from build123d import *

# Parameters (mm, degrees)
F1_DEPTH = 762
F2_R     = 5
F3_DEPTH = 25
F4_R     = 5
F5_DEPTH = 25
F6_R     = 5
F7_DEPTH = 25
F8_R     = 5
F9_DEPTH = 25


with BuildPart() as f1:
    # F0 (on Front) → F1 (new body)
    with BuildSketch(Plane.XZ):
        with BuildLine():
            Line((20.354675, 24.193632), (-17.745325, 24.193632))
            ThreePointArc((-17.745325, 24.193632), (-22.235453, 22.33376), (-24.095325, 17.843632))
            Line((-24.095325, 17.843632), (-24.095325, -20.256368))
            ThreePointArc((-24.095325, -20.256368), (-22.235453, -24.746497), (-17.745325, -26.606368))
            Line((-17.745325, -26.606368), (20.354675, -26.606368))
            ThreePointArc((20.354675, -26.606368), (24.844803, -24.746497), (26.704675, -20.256368))
            Line((26.704675, -20.256368), (26.704675, 17.843632))
            ThreePointArc((26.704675, 17.843632), (24.844803, 22.33376), (20.354675, 24.193632))
        make_face()
        with BuildLine():
            ThreePointArc((-17.745325, 11.493632), (-15.885453, 15.98376), (-11.395325, 17.843632))
            Line((-11.395325, 17.843632), (14.004675, 17.843632))
            ThreePointArc((14.004675, 17.843632), (18.494803, 15.98376), (20.354675, 11.493632))
            Line((20.354675, 11.493632), (20.354675, -13.906368))
            ThreePointArc((20.354675, -13.906368), (18.494803, -18.396497), (14.004675, -20.256368))
            Line((14.004675, -20.256368), (-11.395325, -20.256368))
            ThreePointArc((-11.395325, -20.256368), (-15.885453, -18.396497), (-17.745325, -13.906368))
            Line((-17.745325, -13.906368), (-17.745325, 11.493632))
        make_face(mode=Mode.SUBTRACT)
    extrude(amount=F1_DEPTH)

    # F2 (on face) → F3 (cut)
    with BuildSketch(Plane.YZ.offset(26.704675)):
        with Locations((-15, 9.193632)):
            Circle(F2_R)
        with Locations((-15, -11.606368)):
            Circle(F2_R)
        with Locations((-61.2, 9.193632)):
            Circle(F2_R)
        with Locations((-61.2, -11.606368)):
            Circle(F2_R)
    extrude(amount=-F3_DEPTH, mode=Mode.SUBTRACT)

    # F4 (on face) → F5 (cut)
    with BuildSketch(Plane(origin=(0, 0, -26.606368), x_dir=(1, 0, 0), z_dir=(0, 0, -1))):
        with Locations((11.704675, 15)):
            Circle(F4_R)
        with Locations((-9.095325, 15)):
            Circle(F4_R)
        with Locations((11.704675, 61.2)):
            Circle(F4_R)
        with Locations((-9.095325, 61.2)):
            Circle(F4_R)
    extrude(amount=-F5_DEPTH, mode=Mode.SUBTRACT)

    # F6 (on face) → F7 (cut)
    with BuildSketch(Plane(origin=(0, 0, -26.606368), x_dir=(1, 0, 0), z_dir=(0, 0, -1))):
        with Locations((1.304675, 738.9)):
            Circle(F6_R)
        with Locations((1.304675, 708.9)):
            Circle(F6_R)
    extrude(amount=-F7_DEPTH, mode=Mode.SUBTRACT)

    # F8 (on face) → F9 (cut)
    with BuildSketch(Plane.YZ.offset(26.704675)):
        with Locations((-738.9, -1.206368)):
            Circle(F8_R)
        with Locations((-708.9, -1.206368)):
            Circle(F8_R)
    extrude(amount=-F9_DEPTH, mode=Mode.SUBTRACT)


solid = f1.part
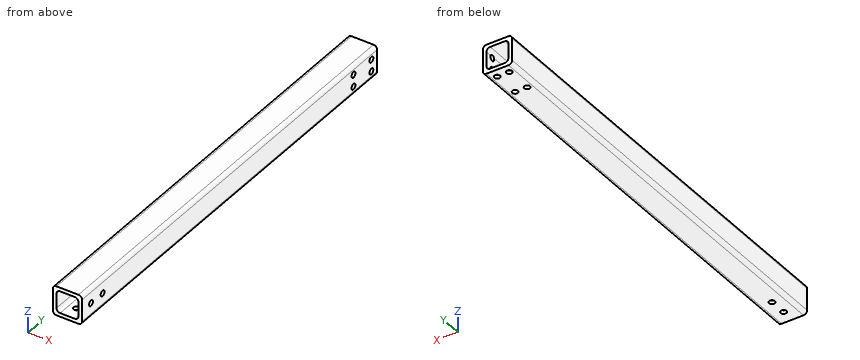
Check sheet for the modelled part. Datum: model origin and axes. Units: mm. Give positions to 0.01 mm unless a question says otherwise; leave off trailing zeros. Write each loop counter-clockwise with the first axis right and the second up, starting at its lowest first coordinate (ties: lowest second). Pieces come first, ordered by that corner, then holes. Notation, with made-up numbers: (36, 47.5) -> (83, 47.5) arc R20 cw to (83, 56.5) -> close; hole circle Ø10 at (0.5, -14.5). An arc over 180 degrees is marked (long way). One line per item, written item: value. Start each with the question number.
Item 1: Gauge pin test, flat end, axial feed: pin 1 (9 mm diameter, centred on y = -61.2, z = -11.61, fed in from +X). Record the tip position at first contact, or that the pin passes through.
Item 2: Section check A-A on y = -344.5. Record the cut outline in (x, z), then the cut area to 3 significant figures.
Item 3: Material ranges on probe 1 along Z at (x, y) = (21.5, -61.2); probe 2 along X at (y, z) = (-67.5, -7); probe 3 along Z at (x, y) = (-9, -170.5), recorded low to high. Write a range as from..to.
Results list:
1. pin 1: x = -17.35
2. outline: (-24.1, -20.26) arc R6.35 ccw to (-17.75, -26.61) -> (20.35, -26.61) arc R6.35 ccw to (26.7, -20.26) -> (26.7, 17.84) arc R6.35 ccw to (20.35, 24.19) -> (-17.75, 24.19) arc R6.35 ccw to (-24.1, 17.84) -> close; hole (-17.75, -13.91) arc R6.35 ccw to (-11.4, -20.26) -> (14, -20.26) arc R6.35 ccw to (20.35, -13.91) -> (20.35, 11.49) arc R6.35 ccw to (14, 17.84) -> (-11.4, 17.84) arc R6.35 ccw to (-17.75, 11.49) -> close
2. area: 1,130 mm²
3. probe 1: -26.5..-16.61, -6.61..4.19, 14.19..24.09
3. probe 2: -24.1..-17.75, 20.35..26.7
3. probe 3: -26.61..-20.26, 17.84..24.19
